Source: CAD feature listing. Evaluate the final solid. Frame: model axes, mm. Give positions to 0.01 mm unless a question says otherwise; leave off trailing zeros. Write each loop counter-clockwise with the first axis right and the second up, starting at its lowest first coordinate (ties: lowest second). Pieces come first, ordered by that corner, then holes. Notation, with made-up numbers: (51.25, -34) -> (67.25, -34) arc R11 cw to (67.25, -15) -> close; hole circle Ø2 at (19, 67). An arc over 180 degrees is marked (long way). Use one line per item in the form item = value. Start each with the question number.
(1) Cut plane B-B, the plane z = 70. Output: boundary loops of the cut face in (x, y), and give its area (3 significant figures).
(2) Material intervals for line 1 along X through (y, z) = (10.75, -70); line 2 along Z through (x, y) = (170, 7.5); line 3 along Z through (x, y) = (2, 16.75), sorted ascending. Write a range as from..to.
(3) Cut plane C-C, the plane x = 0. Output: boundary loops of the cut face in (y, z).
(4) Cut plane A-A, the plane x = -170. Output: boundary loops of the cut face in (y, z), and give its area (3 significant figures).
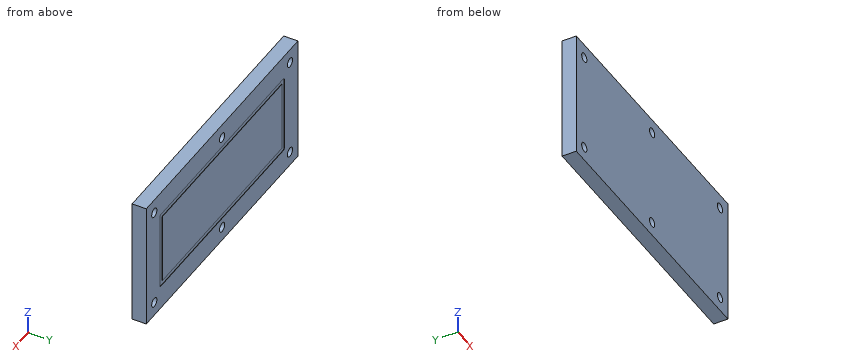
from build123d import *

# Parameters (mm, degrees)
SKETCH1_W           = 380
SKETCH1_H           = 180
BOSS_EXTRUDE1_DEPTH = 20
SKETCH2_R           = 6.5
CUT_EXTRUDE1_DEPTH  = 21
SKETCH3_W           = 300
SKETCH3_H           = 100
CUT_EXTRUDE2_DEPTH  = 0.5


with BuildPart() as part:
    # Sketch1 → Boss-Extrude1 (new body)
    with BuildSketch(Plane(origin=(0, 0, 0), x_dir=(1, 0, 0), z_dir=(0, 1, 0))):
        Rectangle(SKETCH1_W, SKETCH1_H)
    extrude(amount=BOSS_EXTRUDE1_DEPTH)

    # Sketch2 → Cut-Extrude1 (cut, through all)
    with BuildSketch(Plane(origin=(0, 20, 0), x_dir=(1, 0, 0), z_dir=(0, 1, 0))):
        with Locations((-170, 70)):
            Circle(SKETCH2_R)
        with Locations((-170, -70)):
            Circle(SKETCH2_R)
        with Locations((0, -70)):
            Circle(SKETCH2_R)
        with Locations((0, 70)):
            Circle(SKETCH2_R)
        with Locations((170, -70)):
            Circle(SKETCH2_R)
        with Locations((170, 70)):
            Circle(SKETCH2_R)
    extrude(amount=-CUT_EXTRUDE1_DEPTH, mode=Mode.SUBTRACT)

    # Sketch3 → Cut-Extrude2 (cut)
    with BuildSketch(Plane(origin=(0, 20, 0), x_dir=(1, 0, 0), z_dir=(0, 1, 0))):
        with BuildLine():
            Line((-153, -56), (153, -56))
            ThreePointArc((153, -56), (155.121320344, -55.121320344), (156, -53))
            Line((156, -53), (156, 53))
            ThreePointArc((156, 53), (155.121320344, 55.121320344), (153, 56))
            Line((153, 56), (-153, 56))
            ThreePointArc((-153, 56), (-155.121320344, 55.121320344), (-156, 53))
            Line((-156, 53), (-156, -53))
            ThreePointArc((-156, -53), (-155.121320344, -55.121320344), (-153, -56))
        make_face()
        Rectangle(SKETCH3_W, SKETCH3_H, mode=Mode.SUBTRACT)
    extrude(amount=-CUT_EXTRUDE2_DEPTH, mode=Mode.SUBTRACT)


solid = part.part
Geometry says:
q1.outline = (-190, 0) -> (-176.5, 0) -> (-176.5, 20) -> (-190, 20) -> close; (-163.5, 0) -> (-6.5, 0) -> (-6.5, 20) -> (-163.5, 20) -> close; (6.5, 0) -> (163.5, 0) -> (163.5, 20) -> (6.5, 20) -> close; (176.5, 0) -> (190, 0) -> (190, 20) -> (176.5, 20) -> close
q1.area = 6,820 mm^2
q2.line_1 = -190..-176.5, -163.5..-6.5, 6.5..163.5, 176.5..190
q2.line_2 = -90..-76.5, -63.5..63.5, 76.5..90
q2.line_3 = -90..-76.18, -63.82..63.82, 76.18..90
q3.outline = (0, -90) -> (20, -90) -> (20, -76.5) -> (0, -76.5) -> close; (0, -63.5) -> (20, -63.5) -> (20, -56) -> (19.5, -56) -> (19.5, -50) -> (20, -50) -> (20, 50) -> (19.5, 50) -> (19.5, 56) -> (20, 56) -> (20, 63.5) -> (0, 63.5) -> close; (0, 76.5) -> (20, 76.5) -> (20, 90) -> (0, 90) -> close
q4.outline = (0, -90) -> (20, -90) -> (20, -76.5) -> (0, -76.5) -> close; (0, -63.5) -> (20, -63.5) -> (20, 63.5) -> (0, 63.5) -> close; (0, 76.5) -> (20, 76.5) -> (20, 90) -> (0, 90) -> close
q4.area = 3,080 mm^2
